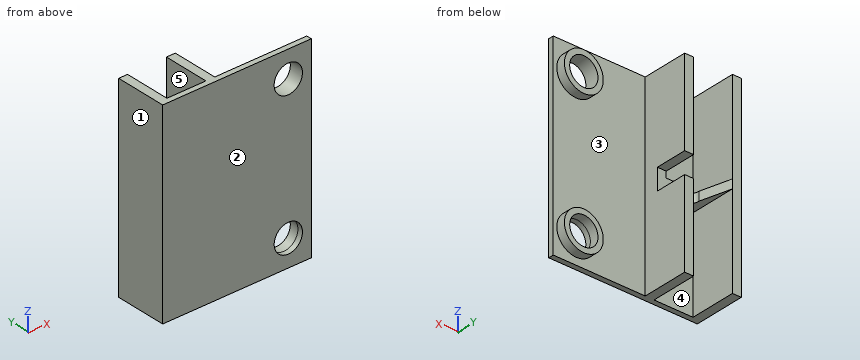
from build123d import *

# Parameters (mm, degrees)
SKETCH1_W                       = 42
SKETCH1_H                       = 55
BOSS_EXTRUDE1_DEPTH             = 1.5
BOSS_EXTRUDE2_REACH             = 29.5
SKETCH2_W                       = 16
SKETCH2_H                       = 13
BOSS_EXTRUDE2_DIRECTION_2_REACH = 29.5
SKETCH3_W                       = 11
SKETCH3_H                       = 13
CUT_EXTRUDE2_DEPTH              = 56
SKETCH6_W                       = 16
SKETCH6_H                       = 13.028292271
BOSS_EXTRUDE3_DEPTH             = 1.25
CUT_EXTRUDE5_DEPTH              = 2.5
SKETCH8_W                       = 6
SKETCH8_H                       = 9
CUT_EXTRUDE6_DEPTH              = 6.5
SKETCH9_R                       = 5.5
SKETCH9_R_2                     = 4
BOSS_EXTRUDE4_DEPTH             = 2.5
SKETCH11_R                      = 4
CUT_EXTRUDE7_DEPTH              = 2.5


with BuildPart() as part:
    # Sketch1 → Boss-Extrude1 (new body)
    with BuildSketch(Plane(origin=(0, 0, 0), x_dir=(1, 0, 0), z_dir=(0, 1, 0))):
        Rectangle(SKETCH1_W, SKETCH1_H)
    extrude(amount=BOSS_EXTRUDE1_DEPTH)

    # Boss-Extrude2: up to this face of the body (flat: up to its plane)
    boss_extrude2_end = Plane(part.part.faces().sort_by_distance((0, 0.75, 27.5))[0])
    # Sketch2 → Boss-Extrude2 (add, up to the picked face)
    with BuildSketch(Plane.XY, mode=Mode.PRIVATE) as boss_extrude2_sk1:
        with Locations((-13, 8)):
            Rectangle(SKETCH2_W, SKETCH2_H)
    boss_extrude2_tool1 = split(extrude(boss_extrude2_sk1.sketch, amount=BOSS_EXTRUDE2_REACH, mode=Mode.PRIVATE), bisect_by=boss_extrude2_end, keep=Keep.BOTH, mode=Mode.PRIVATE)
    add(boss_extrude2_tool1.solids().sort_by_distance((-13, 8, 0))[0])

    # Boss-Extrude2 direction 2: up to this face of the body (flat: up to its plane)
    boss_extrude2_direction_2_end = Plane(part.part.faces().sort_by_distance((0, 0.75, -27.5))[0])
    # Sketch2 → Boss-Extrude2 direction 2 (add, up to the picked face)
    with BuildSketch(Plane.XY, mode=Mode.PRIVATE) as boss_extrude2_direction_2_sk1:
        with Locations((-13, 8)):
            Rectangle(SKETCH2_W, SKETCH2_H)
    boss_extrude2_direction_2_tool1 = split(extrude(boss_extrude2_direction_2_sk1.sketch, amount=-BOSS_EXTRUDE2_DIRECTION_2_REACH, mode=Mode.PRIVATE), bisect_by=boss_extrude2_direction_2_end, keep=Keep.BOTH, mode=Mode.PRIVATE)
    add(boss_extrude2_direction_2_tool1.solids().sort_by_distance((-13, 8, 0))[0])

    # Sketch3 → Cut-Extrude2 (cut, through all)
    with BuildSketch(Plane.XY.offset(27.5)):
        with Locations((-13, 8)):
            Rectangle(SKETCH3_W, SKETCH3_H)
    extrude(amount=-CUT_EXTRUDE2_DEPTH, mode=Mode.SUBTRACT)

    # Sketch6 → Boss-Extrude3 (add, symmetric)
    with BuildSketch(Plane.XY):
        with Locations((-13, 7.985853865)):
            Rectangle(SKETCH6_W, SKETCH6_H)
    extrude(amount=BOSS_EXTRUDE3_DEPTH, both=True)

    # Sketch7 → Cut-Extrude5 (cut)
    with BuildSketch(Plane.XY.offset(1.25)):
        with BuildLine():
            Line((-7.5, 14.5), (-18.5, 14.5))
            Line((-18.5, 14.5), (-16.373292693, 6.010430414))
            ThreePointArc((-16.373292693, 6.010430414), (-13, 2.637137721), (-9.626707307, 6.010430414))
            Line((-9.626707307, 6.010430414), (-7.5, 14.5))
        make_face()
    extrude(amount=-CUT_EXTRUDE5_DEPTH, mode=Mode.SUBTRACT)

    # Sketch8 → Cut-Extrude6 (cut)
    with BuildSketch(Plane(origin=(-5, 0, 0), x_dir=(0, 0, -1), z_dir=(1, 0, 0))):
        with Locations((0, 10)):
            Rectangle(SKETCH8_W, SKETCH8_H)
    extrude(amount=-CUT_EXTRUDE6_DEPTH, mode=Mode.SUBTRACT)

    # Sketch9 → Boss-Extrude4 (add)
    with BuildSketch(Plane(origin=(0, 1.5, 0), x_dir=(1, 0, 0), z_dir=(0, 1, 0))):
        with Locations((14.5, 20)):
            Circle(SKETCH9_R)
        with Locations((14.5, 20)):
            Circle(SKETCH9_R_2, mode=Mode.SUBTRACT)
    boss_extrude4 = extrude(amount=BOSS_EXTRUDE4_DEPTH)

    # Sketch11 → Cut-Extrude7 (cut)
    with BuildSketch(Plane(origin=(0, 1.5, 0), x_dir=(1, 0, 0), z_dir=(0, 1, 0))):
        with Locations((14.5, 20)):
            Circle(SKETCH11_R)
    cut_extrude7 = extrude(amount=-CUT_EXTRUDE7_DEPTH, mode=Mode.SUBTRACT)

    # Mirror1: Boss-Extrude4, Cut-Extrude7 across plane
    add(boss_extrude4.mirror(Plane.XY))
    add(cut_extrude7.mirror(Plane.XY), mode=Mode.SUBTRACT)


solid = part.part
Here's how the part is built. I have some questions about the finished solid (model axes, mm). Face numbers are marked on the shaded views. A direction names the side the tool comes from. Coordinates: 2 decimals unless noted, no trailing zeros. Write each loop counter-clockwise with the first axis right and the second up, starting at its lowest first coordinate (ties: lowest second). Pieces come first, ordered by that corner, then holes.
1) If we section it at A-A (z = 20): List the corners of the cut face in (x, y) for me, plus the area to 4 significant figures.
Filled in:
outline: (-21, 0) - (10.5, 0) - (10.5, 4) - (9, 4) - (9, 1.5) - (-5, 1.5) - (-5, 14.5) - (-7.5, 14.5) - (-7.5, 1.5) - (-18.5, 1.5) - (-18.5, 14.5) - (-21, 14.5) - close; (18.5, 0) - (21, 0) - (21, 1.5) - (20, 1.5) - (20, 4) - (18.5, 4) - close
area: 123.5 mm2
2) Which directions (+Z, -Z, +X, -X, +Y, -Y) give clear straight access to the entire face, cutting with the end or side of a thin tool? Please do the marked faces 4 and 5.
Filled in:
face 4: -Z, +Y
face 5: +Z, +Y
3) I'm going to push flat-ended pins straight in: pin 1 (1.5 mm diameter, centred on x = -13, z = -4.5, fed in from +Y); pin 2 (2.5 mm diameter, centred on x = -8.5, z = -0.5, fed in from +Y); pin 3 (3.5 mm diameter, centred on x = 12, z = 18, fed in from +Y). Where does each tip first touch, or does it pass through?
Filled in:
pin 1: stops at y = 1.5
pin 2: stops at y = 5.5
pin 3: stops at y = 4
4) If I drill on line 1 (Z direction, x = 14.5, y = 2); line 2 (X direction, y = 3.2, z = -20); line 3 (X direction, y = 0.8, z = 20), over which ranges is the centre line in solid material (lowest first)?
Filled in:
line 1: z = -25.5 to -24, -16 to -14.5, 14.5 to 16, 24 to 25.5
line 2: x = -21 to -18.5, -7.5 to -5, 9 to 10.5, 18.5 to 20
line 3: x = -21 to 10.5, 18.5 to 21
5) Thinking about a two-plate mould opening in X: for the marked faces 1, 2 and 3, which applies, +X half, -X half, draft (parallel to the pull), parting line (faces both ways), or undercut?
Filled in:
face 1: -X half
face 2: draft
face 3: undercut
6) If we section it at C-C (y = 8.5): List the corners of the cut face in (x, z) for me.
Filled in:
outline: (-21, -27.5) - (-18.5, -27.5) - (-18.5, -1.25) - (-17, -1.25) - (-17, 1.25) - (-18.5, 1.25) - (-18.5, 27.5) - (-21, 27.5) - close; (-7.5, -27.5) - (-5, -27.5) - (-5, -3) - (-7.5, -3) - close; (-7.5, 3) - (-5, 3) - (-5, 27.5) - (-7.5, 27.5) - close
7) If we section it at D-D (z = -2): List the corners of the cut face in (x, y) for me, plus the area to 4 significant figures.
Filled in:
outline: (-21, 0) - (21, 0) - (21, 1.5) - (-5, 1.5) - (-5, 5.5) - (-7.5, 5.5) - (-7.5, 1.5) - (-18.5, 1.5) - (-18.5, 14.5) - (-21, 14.5) - close
area: 105.5 mm2
8) If we section it at B-B (x = 14.5): List the corners of the cut face in (y, z) for me, plus the area to 3 significant figures.
Filled in:
outline: (0, -27.5) - (1.5, -27.5) - (1.5, -25.5) - (4, -25.5) - (4, -24) - (0, -24) - close; (0, -16) - (4, -16) - (4, -14.5) - (1.5, -14.5) - (1.5, 14.5) - (4, 14.5) - (4, 16) - (0, 16) - close; (0, 24) - (4, 24) - (4, 25.5) - (1.5, 25.5) - (1.5, 27.5) - (0, 27.5) - close
area: 73.5 mm2
